from build123d import *

# Parameters (mm, degrees)
F1_DEPTH = 9.398
F3_DEPTH = 50.292
F4_DEPTH = 25.4
F6_W     = 14.479677
F6_H     = 23.901559
F7_DEPTH = 8.89


with BuildPart() as f1:
    # F0 (on Top) → F1 (new body)
    with BuildSketch(Plane.XY):
        Polygon((-2.924524, -44.697735), (41.606344, -16.593747), (28.638659, 34.442235), (-23.90668, 37.880219), (-43.4138, -11.030972), align=None)
    extrude(amount=F1_DEPTH)

    # F2 (on Top) → F3 (join)
    with BuildSketch(Plane.XY):
        Polygon((-3.621473, -30.167894), (27.572275, -12.766617), (20.662076, 22.27769), (-14.80241, 26.534987), (-29.810468, -5.878166), align=None)
    extrude(amount=F3_DEPTH)

    # F3_face (on face) → F4 (join)
    with BuildSketch(Plane.XY.offset(50.292)):
        Polygon((-29.810468, -5.878166), (-3.621473, -30.167894), (27.572275, -12.766617), (20.662076, 22.27769), (-14.80241, 26.534987), align=None)
    extrude(amount=F4_DEPTH)

    # F6 (on face) → F7 (join)
    with BuildSketch(Plane(origin=(24.117176, 4.755536, 0), x_dir=(-0.193459, 0.981108, 0), z_dir=(0.981108, 0.193459, 0))):
        with Locations((0.480323, 30.59422)):
            Rectangle(F6_W, F6_H)
    extrude(amount=-F7_DEPTH)


solid = f1.part
Here's how the part is built. I have some questions about the finished solid (model axes, mm). A direction names the side the tool comes from. Coordinates: 2 decimals unless noted, no trailing zeros. Loops run counter-clockwise (first coordinate to the right, second up) from the corner with the lowest first, then second, coordinate; pieces in that order, holes last.
1. For P1, Ø1.8, axis at x = 23.5, y = 7.5, coming from the -Z side; P2, Ø5, axis at x = -20.5, z = 55, coming from the +Y side; P3, Ø6, axis at x = 8.5, z = 26.5, coming from the +Y side; P4, Ø2, axis at y = -20, z = 49, coming from the +X side, each with a flat end and sliding along its axis, tell me the tip position at first contact or that it passes through.
2. I need wall thicknesses on L1, parallel to Z at x = 31.5, y = -2; L2, parallel to Y at x = 18, z = 11.5; L3, parallel to X at y = 12, z = 67. Which ranges of each line are inside material? Lowest first, please.
3. Imagine slicing it at A-A, the plane z = 7. Please give me the cut outline in (x, y), and give its area (3 significant figures).
4. Imagine slicing it at B-B, the plane y = 1. Please give me the cut outline in (x, z).
5. Imagine slicing it at D-D, the plane z = 55. Please give me the cut outline in (x, y).
6. For faces 1 (the flat face through (-16.9, -17.85, 42.08)), 2 (the flat face through (8, 25, 9.398)), 3 (the flat face through (11.757, -21.589, 42.081)), 4 (the flat face through (-22.2, 10.56, 42.08)), which set-ups out of +Z, -Z, +X, -X, +Y, -Y let a thin tool reach every point of the face, with its end or its side?
7. Imagine slicing it at C-C, the plane x = -19.5. Please give me the cut outline in (y, z).
Taken from the geometry:
1. P1: stops at z = 0
1. P2: stops at y = 19.63
1. P3: stops at y = 24.1
1. P4: stops at x = 16.4
2. L1: z = 0 to 9.4
2. L2: y = -18.11 to 22.6
2. L3: x = -21.53 to 22.69
3. outline: (-43.41, -11.03) - (-2.92, -44.7) - (41.61, -16.59) - (28.64, 34.44) - (-23.91, 37.88) - close
3. area: 4,770 mm2
4. outline: (-38.62, 0) - (37.14, 0) - (37.14, 9.4) - (24.86, 9.4) - (24.86, 75.69) - (-26.63, 75.69) - (-26.63, 9.4) - (-38.62, 9.4) - close
5. outline: (-29.81, -5.88) - (-3.62, -30.17) - (27.57, -12.77) - (20.66, 22.28) - (-14.8, 26.53) - close
6. face 1: +Z, -X, -Y
6. face 2: +Z
6. face 3: +Z, +X, -Y
6. face 4: +Z, -X, +Y
7. outline: (-30.92, 0) - (37.59, 0) - (37.59, 9.4) - (16.39, 9.4) - (16.39, 75.69) - (-15.44, 75.69) - (-15.44, 9.4) - (-30.92, 9.4) - close
